```python
from build123d import *

# Parameters (mm, degrees)
SKETCH1_R           = 44.45
BOSS_EXTRUDE1_DEPTH = 101.6
CHAMFER1_SIZE       = 12.7
SKETCH2_R           = 3.175
BOSS_EXTRUDE2_DEPTH = 25.4
SKETCH4_R           = 44.45
CUT_EXTRUDE1_DEPTH  = 3.175
SKETCH5_W           = 101.6
SKETCH5_H           = 3.175
BOSS_EXTRUDE4_DEPTH = 88.9
SKETCH6_W           = 38.1
SKETCH6_H           = 7.01009255
BOSS_EXTRUDE5_DEPTH = 88.9
SKETCH7_R           = 3.175
CUT_EXTRUDE2_DEPTH  = 88.9
SKETCH8_R           = 3.175
CUT_EXTRUDE3_DEPTH  = 88.9


with BuildPart() as part:
    # Sketch1 → Boss-Extrude1 (new body)
    with BuildSketch(Plane.XY):
        Circle(SKETCH1_R)
    extrude(amount=BOSS_EXTRUDE1_DEPTH)

    # Chamfer1
    chamfer1_edges = [part.edges().sort_by_distance(p)[0] for p in [
        (-44.45, 0, 101.6),
    ]]
    chamfer(chamfer1_edges, length=CHAMFER1_SIZE)

    # Sketch2 → Boss-Extrude2 (add)
    with BuildSketch(Plane(origin=(0, 0, 0), x_dir=(-1, 0, 0), z_dir=(0, 0, -1))):
        with Locations(Location((0, 0, 0), (0, 0, 180))):
            Circle(SKETCH2_R)
    extrude(amount=BOSS_EXTRUDE2_DEPTH)

    # Sketch3 → Revolve2 (revolve)
    with BuildSketch(Plane(origin=(0, 0, 0), x_dir=(0, 0, -1), z_dir=(1, 0, 0)), mode=Mode.PRIVATE) as revolve2_sk:
        with BuildLine():
            Line((25.4, 0), (50.8, 0))
            Line((50.8, 0), (50.8, 50.8))
            Line((50.8, 50.8), (47.625, 50.8))
            ThreePointArc((47.625, 50.8), (38.1, 41.275), (28.575, 50.8))
            Line((28.575, 50.8), (25.4, 50.8))
            Line((25.4, 50.8), (25.4, 0))
        make_face()
    revolve(revolve2_sk.sketch.rotate(Axis((0, 0, -25.4), (0, 0, -1)), 90), axis=Axis((0, 0, -25.4), (0, 0, -1)))

    # Sketch4 → Cut-Extrude1 (cut)
    with BuildSketch(Plane(origin=(0, 0, -50.8), x_dir=(-1, 0, 0), z_dir=(0, 0, -1))):
        Circle(SKETCH4_R)
    extrude(amount=-CUT_EXTRUDE1_DEPTH, mode=Mode.SUBTRACT)



with BuildPart() as body_2:
    # Sketch5 → Boss-Extrude4 (new body)
    with BuildSketch(Plane.XY):
        with Locations((0, -46.0375)):
            Rectangle(SKETCH5_W, SKETCH5_H)
    extrude(amount=BOSS_EXTRUDE4_DEPTH)


with BuildPart() as part_1:
    add(part.part)

    add(body_2.part)  # Boss-Extrude5 merges body 2
    # Sketch6 → Boss-Extrude5 (add)
    with BuildSketch(Plane.XY.offset(88.9)):
        with Locations((0, -40.944953725)):
            Rectangle(SKETCH6_W, SKETCH6_H)
    extrude(amount=-BOSS_EXTRUDE5_DEPTH)

    # Sketch7 → Cut-Extrude2 (cut)
    with BuildSketch(Plane(origin=(0, -44.45, 0), x_dir=(1, 0, 0), z_dir=(0, 1, 0))):
        with Locations(Location((38.1, -19.05, 0), (0, 0, 180))):
            Circle(SKETCH7_R)
        with Locations(Location((38.1, -69.85, 0), (0, 0, 180))):
            Circle(SKETCH7_R)
    extrude(amount=-CUT_EXTRUDE2_DEPTH, mode=Mode.SUBTRACT)

    # Sketch8 → Cut-Extrude3 (cut)
    with BuildSketch(Plane(origin=(0, -44.45, 0), x_dir=(1, 0, 0), z_dir=(0, 1, 0))):
        with Locations(Location((-38.1, -19.05, 0), (0, 0, 180))):
            Circle(SKETCH8_R)
        with Locations(Location((-38.1, -69.85, 0), (0, 0, 180))):
            Circle(SKETCH8_R)
    extrude(amount=-CUT_EXTRUDE3_DEPTH, mode=Mode.SUBTRACT)


solid = part_1.part
```
Can you work these out from the model? Positions are in its coordinate system, mm. A direction names the side the tool comes from. Round coordinates to 2 decimals unless told otherwise and drop trailing zeros. Order: outer loops, then holes, each group sorted by start corner. A loop starts at its lowest first (then second) coordinate and runs counter-clockwise, first axis right, second up.
(1) If I drill on L1, parallel to X at y = -46, z = 19; L2, parallel to Z at x = -38.1, y = -45.3 (3 decimals); L3, parallel to Z at x = 28, y = -8 (3 decimals), over which ranges is the centre line in solid material (lowest first)?
Results are:
L1: x = -50.8 to -41.27, -34.93 to 34.93, 41.27 to 50.8
L2: z = 0 to 15.875, 22.225 to 66.675, 73.025 to 88.9
L3: z = -47.625 to -25.4, 0 to 101.6
(2) We'd pull the mould along Z, two halves only. Please class faces 1 (the face through (0, 45, -50.8)), 2 (the face through (38.79, -46.02, 66.75)), 3 (the face through (-35, -44.45, 44)): +Z half, -Z half, draft (parallel to the pull), parting line (faces both ways), or undercut.
Results are:
face 1: -Z half
face 2: undercut
face 3: draft
(3) I'm going to push flat-ended pins straight in: pin 1 (8 mm diameter, centred on y = -23, z = 35, fed in from -X); pin 2 (10 mm diameter, centred on x = -38.1, z = 69.85, fed in from -Y) (3 decimals); pin 3 (4 mm diameter, centred on x = 38.1, z = 19.05, fed in from -Y). Where does each tip first touch, or does it pass through?
Results are:
pin 1: stops at x = -40.18
pin 2: stops at y = -47.625
pin 3: stops at y = -25.93
(4) If we section it at B-B (z = 48): Please give me the cut outline in (x, y) (3 decimals), plus the area to 3 significant figures.
Results are:
outline: (-50.8, -47.625) - (50.8, -47.625) - (50.8, -44.45) - (19.05, -44.45) - (19.05, -40.161) arc R44.45 ccw (long way) to (-19.05, -40.161) - (-19.05, -44.45) - (-50.8, -44.45) - close
area: 6,580 mm2
(5) If we section it at C-C (y = 0): Please give me the cut outline in (x, z) (3 decimals).
Results are:
outline: (-50.8, -50.8) - (-44.45, -50.8) - (-44.45, -47.625) - (44.45, -47.625) - (44.45, -50.8) - (50.8, -50.8) - (50.8, -47.625) arc R9.525 cw to (50.8, -28.575) - (50.8, -25.4) - (3.175, -25.4) - (3.175, 0) - (44.45, 0) - (44.45, 88.9) - (31.75, 101.6) - (-31.75, 101.6) - (-44.45, 88.9) - (-44.45, 0) - (-3.175, 0) - (-3.175, -25.4) - (-50.8, -25.4) - (-50.8, -28.575) arc R9.525 cw to (-50.8, -47.625) - close
(6) On a 3-axis mill with a long thin cutter (end or side, diameter ignored), from which of +Z, -Z, +X, -X, +Y, -Y can I reach the whole of each face in a straight line? I mean faces 4 (the face through (1.5, 2.8, -12.5)), 5 (the face through (1, 1, -47.625)), 6 (the face through (-37.41, -46.02, 66.75)), 7 (the face through (19.05, -42, 45)), 8 (the face through (1.68, 44.42, 43.83)). Say none if no direction works.
Results are:
face 4: none
face 5: -Z
face 6: -Y
face 7: +Z, +X
face 8: +Z
(7) If we section it at D-D (x = 23): Count the separate pieces of the cut face and the enclosed holes in it, plus the area to 3 significant figures.
Results are:
separate pieces: 3
enclosed holes: 0
area: 9,540 mm2
(8) If we section it at A-A (x = 0): Please give me the cut outline in (y, z) (3 decimals), plus the area to 3 significant figures.
Results are:
outline: (-50.8, -50.8) - (-44.45, -50.8) - (-44.45, -47.625) - (44.45, -47.625) - (44.45, -50.8) - (50.8, -50.8) - (50.8, -47.625) arc R9.525 cw to (50.8, -28.575) - (50.8, -25.4) - (3.175, -25.4) - (3.175, 0) - (44.45, 0) - (44.45, 88.9) - (31.75, 101.6) - (-31.75, 101.6) - (-44.45, 88.9) - (-47.625, 88.9) - (-47.625, 0) - (-3.175, 0) - (-3.175, -25.4) - (-50.8, -25.4) - (-50.8, -28.575) arc R9.525 cw to (-50.8, -47.625) - close
area: 11,300 mm2
